from build123d import *

# Parameters (mm, degrees)
SKETCH_1_W          = 36
SKETCH_1_H          = 30
EXTRUDE_1_DEPTH     = 8
CUT_EXTRUDE_1_REACH = 26.759
SKETCH_9_W          = 15
SKETCH_9_H          = 20
CHAMFER_1_SIZE      = 1
CHAMFER_2_SIZE      = 1
CHAMFER_3_SIZE      = 1


with BuildPart() as part:
    # 草图1 → 凸台-拉伸1 (new body)
    with BuildSketch(Plane.XY):
        Rectangle(SKETCH_1_W, SKETCH_1_H)
    extrude(amount=EXTRUDE_1_DEPTH)

    # 草图9 → 切除-拉伸1 (cut, up to next)
    with BuildSketch(Plane.XY.offset(8), mode=Mode.PRIVATE) as cut_extrude_1_sk1:
        with Locations((0, 5)):
            Rectangle(SKETCH_9_W, SKETCH_9_H)
    cut_extrude_1_tool1 = extrude(cut_extrude_1_sk1.sketch, amount=-CUT_EXTRUDE_1_REACH, mode=Mode.PRIVATE) & part.part
    add(cut_extrude_1_tool1.solids().sort_by_distance((0, 5, 8))[0], mode=Mode.SUBTRACT)

    # 倒角1
    chamfer_1_edges = [part.edges().sort_by_distance(p)[0] for p in [
        (18, -15, 4),
        (-18, -15, 4),
        (-18, 15, 4),
        (18, 15, 4),
    ]]
    chamfer(chamfer_1_edges, length=CHAMFER_1_SIZE)

    # 倒角2
    chamfer_2_edges = [part.edges().sort_by_distance(p)[0] for p in [
        (-7.5, 15, 4),
        (7.5, 15, 4),
    ]]
    chamfer(chamfer_2_edges, length=CHAMFER_2_SIZE)

    # 倒角3
    chamfer_3_edges = [part.edges().sort_by_distance(p)[0] for p in [
        (7.5, -5, 4),
        (-7.5, -5, 4),
    ]]
    chamfer(chamfer_3_edges, length=CHAMFER_3_SIZE)


solid = part.part
Source: CAD feature listing. Evaluate the final solid. Frame: model axes, mm. A direction names the side the tool comes from. Coordinates: 2 decimals unless noted, no trailing zeros. Order: outer loops, then holes, each group sorted by start corner. A loop starts at its lowest first (then second) coordinate and runs counter-clockwise, first axis right, second up. Notation, with made-up numbers: M 31.5,50.25 L 80.5,50.25 A17 ccw 80.5,61.25 Z; hole C -8.5,-38 d7. An arc over 180 degrees is marked long. Write each question's results on one line, items separated by ' | '. Start each with the question number.
Item 1: Draft query along X for faces 1 (the face through (-7, -4.5, 4.1)), 2 (the face through (0, -6, 8)), 3 (the face through (17.5, 14.5, 3.9)). Return one class per face: pulls with the +X half, pulls with the -X half, needs draft (parallel to the pull), parting line crosses it, or undercut.
Item 2: Set-up query: faces 4 (the face through (8, 14.5, 4.1)), 5 (the face through (0, -6, 0)). Return all of +Z, -Z, +X, -X, +Y, -Y with unobstructed straight access to the full face (end or side cutting, diameter ignored); none if empty.
Item 3: First-contact query: pin 1 Ø4 at (x, z) = (1, 2.5) entering from +Y; pin 2 Ø5 at (x, y) = (-10.5, -4) entering from -Z. Flat tips, straight axial feed; report the tip coordinate or a pass-through.
Item 4: Cut plane B-B (z = 5). Return loops of the section in (x, y).
Item 5: Line query: probe 1 along X at (y, z) = (10.5, 2); probe 2 along X at (y, z) = (-4.5, 7.5); probe 3 along Y at (x, z) = (2, 1.5). Output: solid intervals per line, ascending.
Item 6: Cut plane A-A (y = 5.75). Return loops of the section in (x, z), and give its area (3 significant figures).
Item 7: Cut plane C-C (x = -4.5). Return loops of the section in (y, z).
Checked values:
1) face 1: undercut | face 2: needs draft | face 3: pulls with the +X half
2) face 4: +Z, -Z, +Y | face 5: -Z, +X, -X, +Y, -Y
3) pin 1: stops at y = -5 | pin 2: stops at z = 0
4) outline: M -18,-14 L -17,-15 L 17,-15 L 18,-14 L 18,14 L 17,15 L 8.5,15 L 7.5,14 L 7.5,-4 L 6.5,-5 L -6.5,-5 L -7.5,-4 L -7.5,14 L -8.5,15 L -17,15 L -18,14 Z
5) probe 1: x = -18 to -7.5, 7.5 to 18 | probe 2: x = -18 to -7, 7 to 18 | probe 3: y = -15 to -5
6) outline: M -18,0 L -7.5,0 L -7.5,8 L -18,8 Z; M 7.5,0 L 18,0 L 18,8 L 7.5,8 Z | area: 168 mm2
7) outline: M -15,0 L -5,0 L -5,8 L -15,8 Z
